For this review, take the finished solid that the model builds, in its own axes (mm). Coordinates: 2 decimals unless noted, no trailing zeros. Write each loop counter-clockwise with the first axis right and the second up, starting at its lowest first coordinate (ties: lowest second). Pieces come first, ordered by that corner, then holes. Notation, with made-up numbers: (57.5, -7.5) -> (101.5, -7.5) arc R22 cw to (101.5, 30.5) -> close; hole circle Ø7 at (74.5, 64). An arc over 180 degrees is marked (long way). One line per item, written item: value. Start each with the question number.
1) Add section B-B (z = 1.5). State how many separate pieces and enclosed holes the cut face has, and give its area (3 significant figures).
2) For pin 1 Ø1.2 at (x, z) = (-21.5, 1.5) entering from -Y; pin 2 Ø1 at (y, z) = (43.5, 1) entering from -X; pin 3 Ø1 at (x, z) = (16, 1) entering from +Y, all flat-tipped, find the tip position at first contact; note any pin that passes through.
3) For probe 1 along Y at (x, z) = (-45.5, 0.6); probe 2 along X at (y, z) = (11, 1.8); probe 3 along X at (y, z) = (39.5, 1.4), list the stretches that pass through material, from the lowest coordinate up. Write a range as from..to.
4) Add section A-A (x = -27). State the section outline as (y, z) points.
5) Add section D-D (y = 23.5). State the section outline as (x, z) points.
6) Add section C-C (x = -9). State the section outline as (y, z) points, and give its area (3 significant figures).
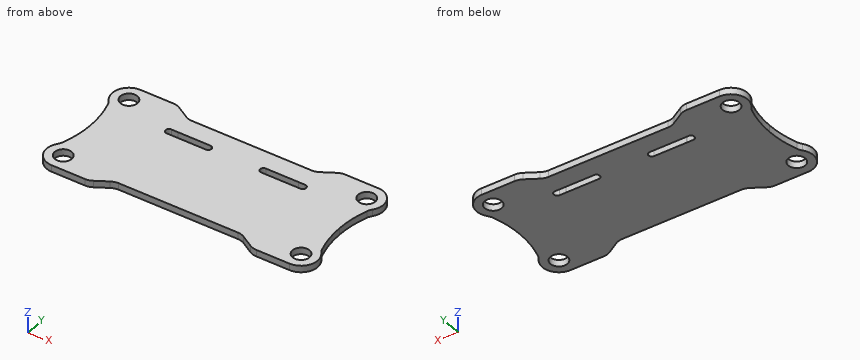
from build123d import *

# Parameters (mm, degrees)
F0_R     = 3.1
F1_DEPTH = 2.4
F3_R     = 5


with BuildPart() as f1:
    # F0 (on Top) → F1 (new body)
    with BuildSketch(Plane.XY):
        with BuildLine():
            ThreePointArc((-49.28070274, 28.4556998014), (-49.8292635669, 22.013644053), (-51.4566855291, 15.7564482751))
            ThreePointArc((-51.4566855291, 15.7564482751), (-52.8417128359, 9.1953601987), (-47.2807049618, 5.4481787499))
            Line((-47.2807049618, 5.4481787499), (-33.8807049618, 5.4481787499))
            Line((-33.8807049618, 5.4481787499), (-27.2140382951, 9.4481787499))
            Line((-27.2140382951, 9.4481787499), (-4.28070274, 9.4481787499))
            Line((-4.28070274, 9.4481787499), (-4.28070274, 11.4481787499))
            Line((-4.28070274, 11.4481787499), (-4.28070274, 45.4481766123))
            Line((-4.28070274, 45.4481766123), (-4.28070274, 47.4481766123))
            Line((-4.28070274, 47.4481766123), (-27.2831063748, 47.4481766123))
            Line((-27.2831063748, 47.4481766123), (-33.9495535553, 51.447781563))
            Line((-33.9495535553, 51.447781563), (-47.2118519247, 51.447781563))
            Line((-47.2118519247, 51.447781563), (-47.3495535553, 51.447781563))
            ThreePointArc((-47.3495535553, 51.447781563), (-52.8586646481, 47.6586835568), (-51.4406336464, 41.1244080183))
            ThreePointArc((-51.4406336464, 41.1244080183), (-49.8251900555, 34.8889789679), (-49.28070274, 28.4707419045))
            Line((-49.28070274, 28.4707419045), (-49.28070274, 28.4556998014))
        make_face()
        with Locations((-47.2807049618, 11.4481787499)):
            Circle(F0_R, mode=Mode.SUBTRACT)
        with Locations((-47.28070274, 45.4481766123)):
            Circle(F0_R, mode=Mode.SUBTRACT)
        with BuildLine():
            Line((-28.4305080615, 40.4512316858), (-26.08070274, 40.4481766123))
            Line((-26.08070274, 40.4481766123), (-14.28070274, 40.4481766123))
            ThreePointArc((-14.28070274, 40.4481766123), (-13.0807048557, 39.2481744965), (-14.2807069714, 38.0481766123))
            Line((-14.2807069714, 38.0481766123), (-26.0736386877, 38.0481974045))
            Line((-26.0736386877, 38.0481974045), (-26.0918883742, 38.0482287461))
            Line((-26.0918883742, 38.0482287461), (-28.4716546856, 38.0523157045))
            ThreePointArc((-28.4716546856, 38.0523157045), (-29.6805192393, 39.2728612272), (-28.4305080615, 40.4512316858))
        make_face(mode=Mode.SUBTRACT)
    extrude(amount=F1_DEPTH)

    # F2: F1 across face


with BuildPart() as f1_1:
    add(f1.part)
    add(f1.part.mirror(Plane(origin=(-4.28070274, 28.4481776811, 1.2), x_dir=(0, 1, 0), z_dir=(1, 0, 0))))

    # F3
    f3_edges = [f1_1.edges().sort_by_distance(p)[0] for p in [
        (-33.949554, 51.447782, 1.2),
        (-27.283106, 47.448177, 1.2),
        (18.721701, 47.448177, 1.2),
        (25.388148, 51.447782, 1.2),
        (-33.880705, 5.448179, 1.2),
        (-27.214038, 9.448179, 1.2),
        (18.652633, 9.448179, 1.2),
        (25.319299, 5.448179, 1.2),
        (-51.456686, 15.756448, 1.2),
        (-51.440634, 41.124408, 1.2),
        (42.89528, 15.756448, 1.2),
        (42.879228, 41.124408, 1.2),
    ]]
    fillet(f3_edges, radius=F3_R)


solid = f1_1.part
Numbers:
1. separate pieces: 1
1. enclosed holes: 6
1. area: 3,680 mm²
2. pin 1: y = 9.45
2. pin 2: x = -53.1
2. pin 3: y = 47.45
3. probe 1: 5.45..8.91, 13.99..42.91, 47.99..51.45
3. probe 2: -53.26..-50.35, -44.21..35.65, 41.79..44.7
3. probe 3: -50.91..-29.65, -13.11..4.55, 21.09..42.35
4. outline: (9.31, 0) -> (38.05, 0) -> (38.05, 2.4) -> (9.31, 2.4) -> close; (40.45, 0) -> (47.57, 0) -> (47.57, 2.4) -> (40.45, 2.4) -> close
5. outline: (-49.6, 0) -> (41.04, 0) -> (41.04, 2.4) -> (-49.6, 2.4) -> close
6. outline: (9.45, 0) -> (47.45, 0) -> (47.45, 2.4) -> (9.45, 2.4) -> close
6. area: 91.2 mm²
